Print and shaded views of the part. All mm, measured from the part's lowest x, y and z. Round coordinates to 2 decimals unless told otherwise and drop trailing zeros. Order: outer loops, then holes, each group sorted by start corner. A loop starts at its lowest first (then second) coordinate and runs counter-clockwise, first axis right, second up. Notation, with made-up numbers: M 75,-11 L 130,-11 A14 ccw 130,9 Z; hole C 46.25,-25 d1. An arc over 180 degrees is marked long. Write each question's results on one line, items separated by ' | '. Start each with the question number.
1. Two-plate mould, pull along X, no slides. Class the marked faces 1, 2 and 3: +X half, -X half, draft (parallel to the pull), parting line (faces both ways), or undercut.
2. Probe L1, parallel to Y at x = 50, z = 255; L2, parallel to X at y = 48, z = 30; L3, parallel to Z at x = 69, y = 24.5. List the from-to ranges inside material, lowest first. Write a range as [from, to].
3. Band-saw the part on A-A, the plane x = 50. List the corners of the cut face in (y, z).
4. Band-saw the part on C-C, the plane z = 51. List the corners of the cut face in (x, y).
5. Band-saw the part on B-B, the plane y = 50. List the corners of the cut face in (x, z), then the cut area to 3 significant figures.
6. Band-saw the part on D-D, the plane z = 227.5. List the corners of the cut face in (x, y).
7. Drop flat-ended pins along their axis: pin 1 Ø2 at (y, z) = (13.5, 231.5) entering from +X; pin 2 Ø5 at (x, z) = (47.5, 277.5) entering from -Y; pin 3 Ø2 at (y, z) = (65.5, 425) entering from -X. Give the stop position or say it passes through.
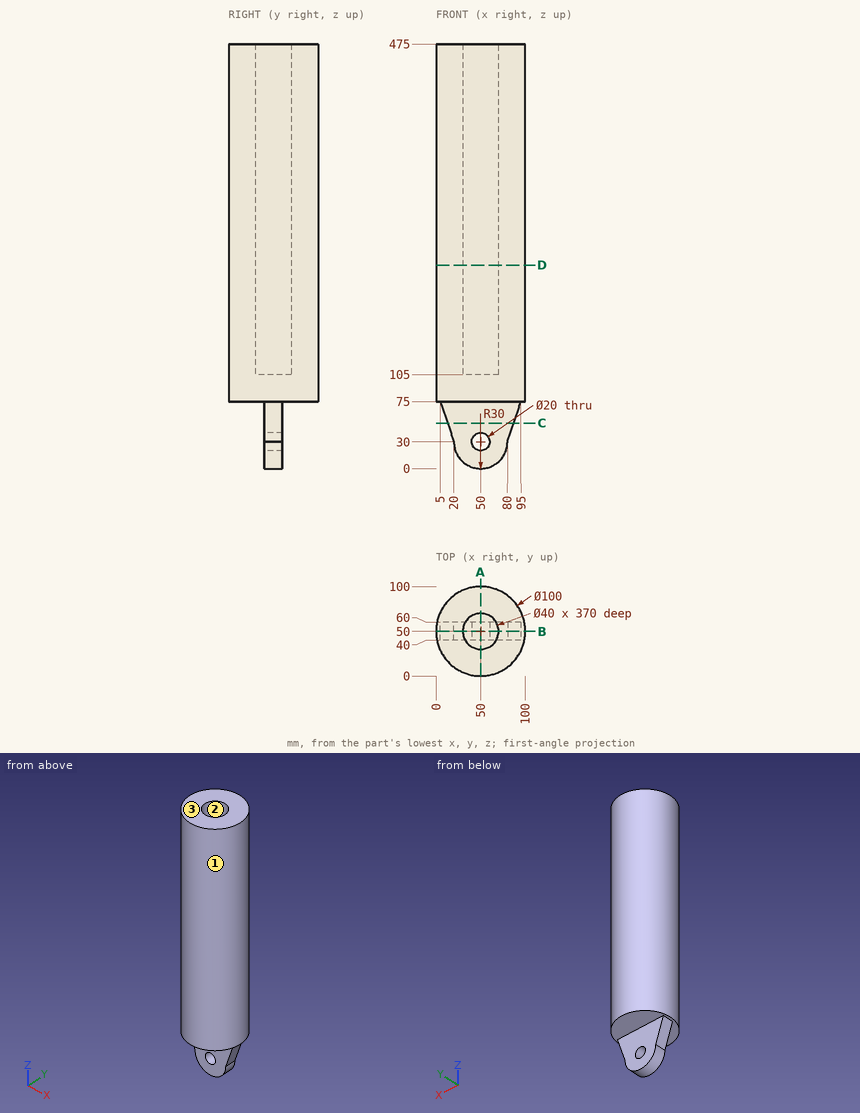
Solution:
1) face 1: parting line | face 2: undercut | face 3: draft
2) L1: [0, 30], [70, 100] | L2: [20, 40], [60, 80] | L3: [75, 475]
3) outline: M 0,75 L 40,75 L 40,40 L 60,40 L 60,75 L 100,75 L 100,475 L 70,475 L 70,105 L 30,105 L 30,475 L 0,475 Z; M 40,0 L 60,0 L 60,20 L 40,20 Z
4) outline: M 13,40 L 87,40 L 87,60 L 13,60 Z
5) outline: M 0,75 L 5,75 L 20,30 A30 ccw 80,30 L 95,75 L 100,75 L 100,475 L 70,475 L 70,105 L 30,105 L 30,475 L 0,475 Z; hole C 50,30 d20 | area: 29,700 mm^2
6) outline: C 50,50 d100; hole C 50,50 d40
7) pin 1: x = 85.21 | pin 2: y = 0 | pin 3: x = 2.15
